Verification items for the finished model (mm, model axes). Face numbers are marked on the shaded views. A direction names the side the tool comes from. Give positions to 0.01 mm unless a question says otherwise; leave off trailing zeros. Write each loop counter-clockwise with the first axis right and the second up, starting at its lowest first coordinate (ties: lowest second). Pieces come first, ordered by that corner, then holes. Notation, with made-up numbers: (21.5, 64) - (74.5, 64) arc R29 ccw to (74.5, 95) - close; hole circle Ø3 at (33.5, 25.25). An arc over 180 degrees is marked (long way). Answer as a JSON object with one key per item and string values. Group by question number.
Item 1: Tool access check on the marked faces 1, 2, 3, 4 and 5. Record the directions out of +Z, -Z, +X, -X, +Y, -Y that give a thin tool (end or side, any length) a straight path to the whole face; none if there is none.
Item 2: Sectioned sample at A-A, the plane x = 27. Record the boundary of the cut face in (y, z).
Item 3: Sectioned sample at D-D, the plane x = -25.4. Record the boundary of the cut face in (y, z).
Item 4: Draft check along Z on the marked faces 6, 7 and 8. Enter one of: +Z half, -Z half, draft (parallel to the pull), parting line (faces both ways), or undercut.
Item 5: Scan lines: line 1 along Y through (x, z) = (-25, -7); line 2 along X through (y, z) = (-12.5, -6.5); line 3 along X through (y, z) = (-25, -5). Record each from-to range of solid material in increasing order. Write a range as [from, to].
Item 6: Sectioned sample at C-C, the plane z = -8. Record the boundary of the cut face in (x, y) (3 decimals).
Item 7: Sectioned sample at B-B, the plane y = -23. Record the boundary of the cut face in (x, z), and give its area (3 significant figures).
Item 8: Go/stop test with flat-tipped pins: pin 1 (7.5 mm diameter, centred on y = -16.5, z = 37.5, fed in from +X); pin 2 (13 mm diameter, centred on x = 31.5, y = -7, fed in from -Z); pin 3 (16 mm diameter, centred on x = -25.4, y = -15.875, fed in from +Z); pin 4 (4 mm diameter, centred on x = 26.5, y = -4, fed in from -Z). Record where each tip stops, or that it passes through.
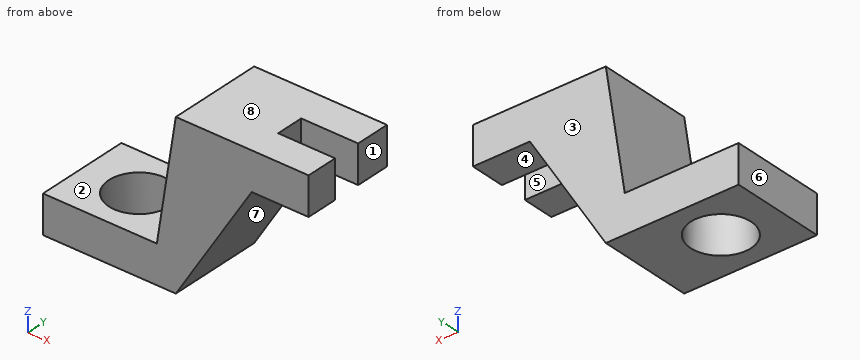
```python
from build123d import *

# Parameters (mm, degrees)
F1_DEPTH = 31.75
F2_R     = 10.096628
F3_DEPTH = 15.748
F4_W     = 19.05
F4_H     = 9.336647
F5_DEPTH = 12.7


with BuildPart() as f1:
    # F0 (on Front) → F1 (new body)
    with BuildSketch(Plane.XZ):
        Polygon((-6.35, 0), (-44.45, 0), (-44.45, -12.7), (0, -12.7), (25.4, 28.448), (44.45, 28.448), (44.45, 41.148), (0, 41.148), align=None)
    extrude(amount=F1_DEPTH)

    # F2 (on face) → F3 (cut)
    with BuildSketch(Plane.XY):
        with Locations((-25.4, -15.875)):
            Circle(F2_R)
    extrude(amount=-F3_DEPTH, mode=Mode.SUBTRACT)

    # F4 (on face) → F5 (cut)
    with BuildSketch(Plane.XY.offset(41.148)):
        with Locations((34.925, -16.351854)):
            Rectangle(F4_W, F4_H)
    extrude(amount=-F5_DEPTH, mode=Mode.SUBTRACT)


solid = f1.part
```
Geometry check:
{
 "1": {"face 1": "+Z, -Z, +X, +Y, -Y", "face 2": "+Z, -X, +Y, -Y", "face 3": "+Z, -Z, +X, -X, +Y", "face 4": "-Z, +X, +Y, -Y", "face 5": "+Z, -Z, +X"},
 "2": {"outline": "(-31.75, 28.45) - (-21.02, 28.45) - (-21.02, 41.15) - (-31.75, 41.15) - close; (-11.68, 28.45) - (0, 28.45) - (0, 41.15) - (-11.68, 41.15) - close"},
 "3": {"outline": "(-31.75, -12.7) - (-25.97, -12.7) - (-25.97, 0) - (-31.75, 0) - close; (-5.78, -12.7) - (0, -12.7) - (0, 0) - (-5.78, 0) - close"},
 "4": {"face 6": "draft", "face 7": "-Z half", "face 8": "+Z half"},
 "5": {"line 1": "[-31.75, -25.96], [-5.79, 0]", "line 2": "[-44.45, -34.92], [-15.88, 3.83]", "line 3": "[-44.45, -29.72], [-21.08, 4.75]"},
 "6": {"outline": "(-44.45, -31.75) - (2.901, -31.75) - (2.901, 0) - (-44.45, 0) - close; hole circle Ø20.193 at (-25.4, -15.875)"},
 "7": {"outline": "(-44.45, -12.7) - (-32.55, -12.7) - (-32.55, 0) - (-44.45, 0) - close; (-18.25, -12.7) - (0, -12.7) - (25.4, 28.45) - (44.45, 28.45) - (44.45, 41.15) - (0, 41.15) - (-6.35, 0) - (-18.25, 0) - close", "area": "1,600 mm^2"},
 "8": {"pin 1": "x = 25.4", "pin 2": "z = 27.8", "pin 3": "through", "pin 4": "z = 26.99"}
}
